For this review, take the finished solid that the model builds, in its own axes (mm). A direction names the side the tool comes from. Coordinates: 2 decimals unless noted, no trailing zeros. Loops run counter-clockwise (first coordinate to the right, second up) from the corner with the lowest first, then second, coordinate; pieces in that order, holes last.
```python
from build123d import *

# Parameters (mm, degrees)
BOSS_EXTRUDE1_DEPTH      = 55
BOSS_EXTRUDE1_DEPTH_BACK = 10
SKETCH1_R                = 37.5
SKETCH2_R                = 16
CUT_EXTRUDE1_DEPTH       = 16
SKETCH3_R                = 16
CUT_EXTRUDE2_DEPTH       = 2.5
SKETCH6_R                = 8.9296875
CUT_EXTRUDE3_DEPTH       = 23
SKETCH7_R                = 37.5
CUT_EXTRUDE4_DEPTH       = 15.35
SKETCH9_R                = 3.302
BOLT_HOLES_DEPTH         = 73.647247023


with BuildPart() as part:
    # Sketch1 → Boss-Extrude1 (new, two sides: drawn at the far end of the back side and taken through both)
    with BuildSketch(Plane.XY.offset(-BOSS_EXTRUDE1_DEPTH_BACK)):
        Circle(SKETCH1_R)
    extrude(amount=BOSS_EXTRUDE1_DEPTH + BOSS_EXTRUDE1_DEPTH_BACK)

    # Sketch2 → Cut-Extrude1 (cut)
    with BuildSketch(Plane.XY.offset(55)):
        Circle(SKETCH2_R)
    extrude(amount=-CUT_EXTRUDE1_DEPTH, mode=Mode.SUBTRACT)

    # Sketch3 → Cut-Extrude2 (cut)
    with BuildSketch(Plane.XY.offset(39)):
        Circle(SKETCH3_R)
    extrude(amount=-CUT_EXTRUDE2_DEPTH, mode=Mode.SUBTRACT)

    # Sketch4 → Aortic Root (revolve, cut)
    with BuildSketch(Plane(origin=(0, 0, 0), x_dir=(0, 0, -1), z_dir=(1, 0, 0)), mode=Mode.PRIVATE) as aortic_root_sk:
        with BuildLine():
            Line((-19.46, 12), (-19.46, 0))
            Line((-19.46, 0), (-36.5, 0))
            Line((-36.5, 0), (-36.5, 12))
            add(Edge.make_bspline(
                [(-36.5, 12), (-27.947018525, 19.440766671), (-19.46, 12)],
                knots=[0, 0, 0, 1, 1, 1], degree=2))
        make_face()
    revolve(aortic_root_sk.sketch.rotate(Axis((0, 0, 19.46), (0, 0, 1)), 270), axis=Axis((0, 0, 19.46), (0, 0, 1)), mode=Mode.SUBTRACT)

    # Sketch6 → Cut-Extrude3 (cut)
    with BuildSketch(Plane(origin=(0, 0, -10), x_dir=(-1, 0, 0), z_dir=(0, 0, -1))):
        Circle(SKETCH6_R)
    extrude(amount=-CUT_EXTRUDE3_DEPTH, mode=Mode.SUBTRACT)

    # Sketch7 → Cut-Extrude4 (cut)
    with BuildSketch(Plane.XY.offset(55)):
        Circle(SKETCH7_R)
    extrude(amount=-CUT_EXTRUDE4_DEPTH, mode=Mode.SUBTRACT)

    # Sketch9 → Bolt holes (cut, through all)
    with BuildSketch(Plane(origin=(0, 0, -10), x_dir=(-1, 0, 0), z_dir=(0, 0, -1))):
        with Locations((0, -27.5)):
            Circle(SKETCH9_R)
        with Locations((-19.445436483, -19.445436483)):
            Circle(SKETCH9_R)
        with Locations((-27.5, 0)):
            Circle(SKETCH9_R)
        with Locations((-19.445436483, 19.445436483)):
            Circle(SKETCH9_R)
        with Locations((0, 27.5)):
            Circle(SKETCH9_R)
        with Locations((19.445436483, 19.445436483)):
            Circle(SKETCH9_R)
        with Locations((27.5, 0)):
            Circle(SKETCH9_R)
        with Locations((19.445436483, -19.445436483)):
            Circle(SKETCH9_R)
    extrude(amount=-BOLT_HOLES_DEPTH, mode=Mode.SUBTRACT)

    # Sketch12 → Cut-Revolve1 (revolve, cut)
    with BuildSketch(Plane(origin=(0, 0, 0), x_dir=(1, 0, 0), z_dir=(0, 1, 0))):
        Polygon((0, -19.46), (0, -13), (8.9296875, -13), (12, -19.46), align=None)
    revolve(axis=Axis((0, 0, 19.46), (0, 0, -1)), mode=Mode.SUBTRACT)


solid = part.part
```
Q1. Consider section A-A (y = -18). State the section outline as (x, z) points, then the cut area to 3 significant figures.
Q2. Machinability: for faces 5 (the face through (16.296, -18.454, 14.477)), 6 (the face through (-3.47, -15.62, 38.1)), which of the approach directions +Z, -Z, +X, -X, +Y, -Y give a long, thin tool a straight path to every point of the face, cutting with its end or side? Answer none if there is none.
Q3. Consider section B-B (z = -6). Count the separate pieces of the cut face and the enclosed holes in it, then the cut area to 3 significant figures.
Q4. For pin 1 Ø8 at (x, z) = (21, 1.5) entering from -Y; pin 2 Ø12 at (x, z) = (-27.5, -5) entering from -Y; pin 3 Ø4 at (x, z) = (22.5, 14.5) entering from +Y; pin 4 Ø5.5 at (x, y) = (-27.5, 0) entering from +Z, all flat-tipped, find the tip position at first contact; note any pin that passes through.
Q5. Consider section C-C (x = -29). State the section outline as (y, z) points, then the cut area to 3 significant figures.
Q6. The part is to be moulded in two halves that separate along X. For faces 1 (the face through (16.142, 0.525, 39.65)), 2 (the face through (-30.65, 0.99, 14.48)), 3 (the face through (-4.88, 37.18, 14.48)), 4 (the face through (-1.19, -9.04, 13.4)), say which applies: +X half, -X half, draft (parallel to the pull), parting line (faces both ways), or undercut.
Q7. Wall thickness on probe 1 along Y at (x, z) = (0, 4); probe 2 along X at (y, z) = (-19, 20); probe 3 along X at (y, z) = (-3, 24.5): over which ranges is each line inside the solid? List them lowest first.
Q8. Consider section D-D (y = -27.5). State the section outline as (x, z) points, then the cut area to 3 significant figures.
Model answer:
1. outline: (-32.9, -10) - (-22.41, -10) - (-22.41, 39.65) - (-32.9, 39.65) - close; (-16.48, -10) - (16.48, -10) - (16.48, 39.65) - (-16.48, 39.65) - close; (22.41, -10) - (32.9, -10) - (32.9, 39.65) - (22.41, 39.65) - close
1. area: 2,680 mm2
2. face 5: +Z, -Z
2. face 6: +Z
3. separate pieces: 1
3. enclosed holes: 9
3. area: 3,890 mm2
4. pin 1: stops at y = -33.43
4. pin 2: stops at y = -30.72
4. pin 3: stops at y = 31.4
4. pin 4: passes through
5. outline: (-23.77, -10) - (-2.94, -10) - (-2.94, 39.65) - (-23.77, 39.65) - close; (2.94, -10) - (23.77, -10) - (23.77, 39.65) - (2.94, 39.65) - close
5. area: 2,070 mm2
6. face 1: draft
6. face 2: undercut
6. face 3: parting line
6. face 4: undercut
7. probe 1: y = -37.5 to -30.8, -24.2 to -8.93, 8.93 to 24.2, 30.8 to 37.5
7. probe 2: x = -32.33 to -22.72, -16.17 to 16.17, 22.72 to 32.33
7. probe 3: x = -37.38 to -28.88, -26.12 to -14.8, 14.8 to 26.12, 28.88 to 37.38
8. outline: (-25.5, -10) - (-3.3, -10) - (-3.3, 39.65) - (-25.5, 39.65) - close; (3.3, -10) - (25.5, -10) - (25.5, 39.65) - (3.3, 39.65) - close
8. area: 2,200 mm2
